Build history of the part. All positions in model axes, mm. A direction names the side the tool comes from. Round coordinates to 2 decimals unless told otherwise and drop trailing zeros. Write each loop counter-clockwise with the first axis right and the second up, starting at its lowest first coordinate (ties: lowest second). Pieces come first, ordered by that corner, then holes.
from build123d import *

# Parameters (mm, degrees)
BOSS_EXTRU_1_DEPTH = 102.5


with BuildPart() as part:
    # Esquisse2 → Boss.-Extru.1 (new body)
    with BuildSketch(Plane(origin=(0, 0, 0), x_dir=(0, 0, -1), z_dir=(1, 0, 0))):
        with BuildLine():
            Line((20.175844181, 57.796560731), (20.175844181, 0))
            Line((20.175844181, 0), (18.175844181, 0))
            Line((18.175844181, 0), (18.175844181, 57.719847418))
            add(Edge.make_bspline(
                [(-7.816037555, 87.197675328), (1.458199142, 84.486674845), (11.235554116, 76.513419425), (17.493683513, 66.237213452), (18.175844181, 57.719847418)],
                knots=[0.581934289, 0.581934289, 0.581934289, 0.73870893, 0.843225358, 1, 1, 1], degree=2))
            Line((-7.816037555, 87.197675328), (-7.259494569, 89.118680248))
            add(Edge.make_bspline(
                [(20.175844181, 57.796560731), (18.360004181, 81.6963399), (-7.259494569, 89.118680248)],
                knots=[0.58124873, 0.58124873, 0.58124873, 1, 1, 1], degree=2))
        make_face()
    extrude(amount=BOSS_EXTRU_1_DEPTH)


solid = part.part
1) Which spindle directions (+Z, -Z, +X, -X, +Y, -Y) get a long thin tool onto all of the face, cutting with end or side? Do faces 1 (the flat face through (102.5, 48, -19)), 2 (the flat face through (51, 28, -18.176)). Say none if no direction does.
Results:
face 1: +Z, -Z, +X, +Y, -Y
face 2: +Z, +X, -X, -Y
2) Slice it at A-A (y = 16.5). Write the cut outline in (x, z).
Results:
outline: (0, -20.18) - (102.5, -20.18) - (102.5, -18.18) - (0, -18.18) - close
3) Pin check, flat tips, straight feed: pin 1 Ø12 at (x, y) = (59.5, 13.5) entering from +Z; pin 2 Ø3 at (x, y) = (92, 71) entering from -Z; pin 3 Ø3 at (x, z) = (59, -1.5) entering from -Y. Stop position of each tip, or through.
Results:
pin 1: stops at z = -18.18
pin 2: stops at z = -17.46
pin 3: stops at y = 82.68
4) Wall check: L1, parallel to Z at x = 88, y = 55; L2, parallel to Z at x = 69, y = 63.5; L3, parallel to Y at x = 93.5, z = -15.25. Give the ranges that are in metal, low to high.
Results:
L1: z = -20.18 to -18.18
L2: z = -19.35 to -17.3
L3: y = 69.56 to 73.76
